Design review of the part built by this model. Coordinates are the model's own, in mm. A direction names the side the tool comes from. Give positions to 0.01 mm unless a question says otherwise; leave off trailing zeros. Loops run counter-clockwise (first coordinate to the right, second up) from the corner with the lowest first, then second, coordinate; pieces in that order, holes last. Notation, with made-up numbers: (42, 61) -> (77, 61) arc R19 ccw to (77, 92) -> close; hole circle Ø9 at (-14, 84). An arc over 180 degrees is marked (long way). Answer in a Markdown table with one row per item. Add a question column.
(1) For pin 1 (3 mm diameter, centred on x = 3, y = 7.5, fed in from -Z), flat-tipped, find the tip position at first contact; note if it passes through.
(2) Draft analysis for pull direction X (two halves, no side actions). For faces 1 (the flat face through (0, -4, 5)), 2 (the cylindrical face through (4.686, 7.279, 5.183)), 3 (the cylindrical face through (4.686, 7.279, -5.316)), 4 (the flat face through (3, 10, -5)), state which applies: +X half, -X half, draft (parallel to the pull), parting line (faces both ways), or undercut.
(3) Consider section A-A on y = 7.5. Write out the cut boundary in (x, z), then the cut area to 3 significant figures.
(4) For faces 5 (the flat face through (6, -4, 5)), 6 (the flat face through (2.29, 9.23, -0.5)), list the 3-axis set-ups (+Z, -Z, +X, -X, +Y, -Y) from which the entire face can be reached by the end or side of a thin tool; tool diameter is ignored.
(5) For line 1 (Z direction, x = 1.2, y = 8.5); line 2 (Z direction, x = 2.6, y = 0); line 3 (X direction, y = 7.5, z = 5.75), list the stretches that pass through material, from the lowest coordinate up.
(6) Consider section D-D on y = -3.25. Write out the cut boundary in (x, z).
(7) Consider section B-B on x = 3. Write out the cut boundary in (y, z), then the cut area to 3 significant figures.
(8) Consider section C-C on z = 3.75. Write out the cut boundary in (x, y).
from build123d import *

# Parameters (mm, degrees)
BOSS_EXTRUDE1_DEPTH = 6
SKETCH2_R           = 1.7
CUT_EXTRUDE1_DEPTH  = 24.151673806


with BuildPart() as part:
    # Sketch1 → Boss-Extrude1 (new body)
    with BuildSketch(Plane(origin=(0, 0, 0), x_dir=(0, 0, -1), z_dir=(1, 0, 0))):
        with BuildLine():
            Line((-0.5, 5.175905718), (-0.5, 10))
            Line((-0.5, 10), (-10, 10))
            Line((-10, 10), (-10, -10))
            Line((-10, -10), (10, -10))
            Line((10, -10), (10, 10))
            Line((10, 10), (0.5, 10))
            Line((0.5, 10), (0.5, 5.175905718))
            ThreePointArc((0.5, 5.175905718), (3.849675311, 3.495711659), (5.2, 0))
            ThreePointArc((5.2, 0), (-3.495711659, -3.849675311), (-0.5, 5.175905718))
        make_face()
    extrude(amount=BOSS_EXTRUDE1_DEPTH)

    # Sketch2 → Cut-Extrude1 (cut, through all)
    with BuildSketch(Plane(origin=(0, 0, -10), x_dir=(-1, 0, 0), z_dir=(0, 0, -1))):
        with Locations(Location((-3, 7.5, 0), (0, 0, 90))):
            Circle(SKETCH2_R)
    extrude(amount=-CUT_EXTRUDE1_DEPTH, mode=Mode.SUBTRACT)


solid = part.part
Values follow:
| question | item | result |
|---|---|---|
| 1 | pin 1 | through |
| 2 | face 1 | -X half |
| 2 | face 2 | undercut |
| 2 | face 3 | undercut |
| 2 | face 4 | draft |
| 3 | outline | (0, -10) -> (1.3, -10) -> (1.3, -0.5) -> (0, -0.5) -> close; (0, 0.5) -> (1.3, 0.5) -> (1.3, 10) -> (0, 10) -> close; (4.7, -10) -> (6, -10) -> (6, -0.5) -> (4.7, -0.5) -> close; (4.7, 0.5) -> (6, 0.5) -> (6, 10) -> (4.7, 10) -> close |
| 3 | area | 49.4 mm2 |
| 4 | face 5 | +Z, -Z, +X, +Y, -Y |
| 4 | face 6 | +X, -X, +Y |
| 5 | line 1 | -10 to -0.5, 0.5 to 10 |
| 5 | line 2 | -10 to -5.2, 5.2 to 10 |
| 5 | line 3 | 0 to 1.3, 4.7 to 6 |
| 6 | outline | (0, -10) -> (6, -10) -> (6, -4.06) -> (0, -4.06) -> close; (0, 4.06) -> (6, 4.06) -> (6, 10) -> (0, 10) -> close |
| 7 | outline | (-10, -10) -> (5.8, -10) -> (5.8, -0.5) -> (5.18, -0.5) arc R5.2 cw (long way) to (5.18, 0.5) -> (5.8, 0.5) -> (5.8, 10) -> (-10, 10) -> close; (9.2, -10) -> (10, -10) -> (10, -0.5) -> (9.2, -0.5) -> close; (9.2, 0.5) -> (10, 0.5) -> (10, 10) -> (9.2, 10) -> close |
| 7 | area | 246 mm2 |
| 8 | outline | (0, -10) -> (6, -10) -> (6, -3.6) -> (0, -3.6) -> close; (0, 3.6) -> (6, 3.6) -> (6, 10) -> (0, 10) -> close; hole circle Ø3.4 at (3, 7.5) |
